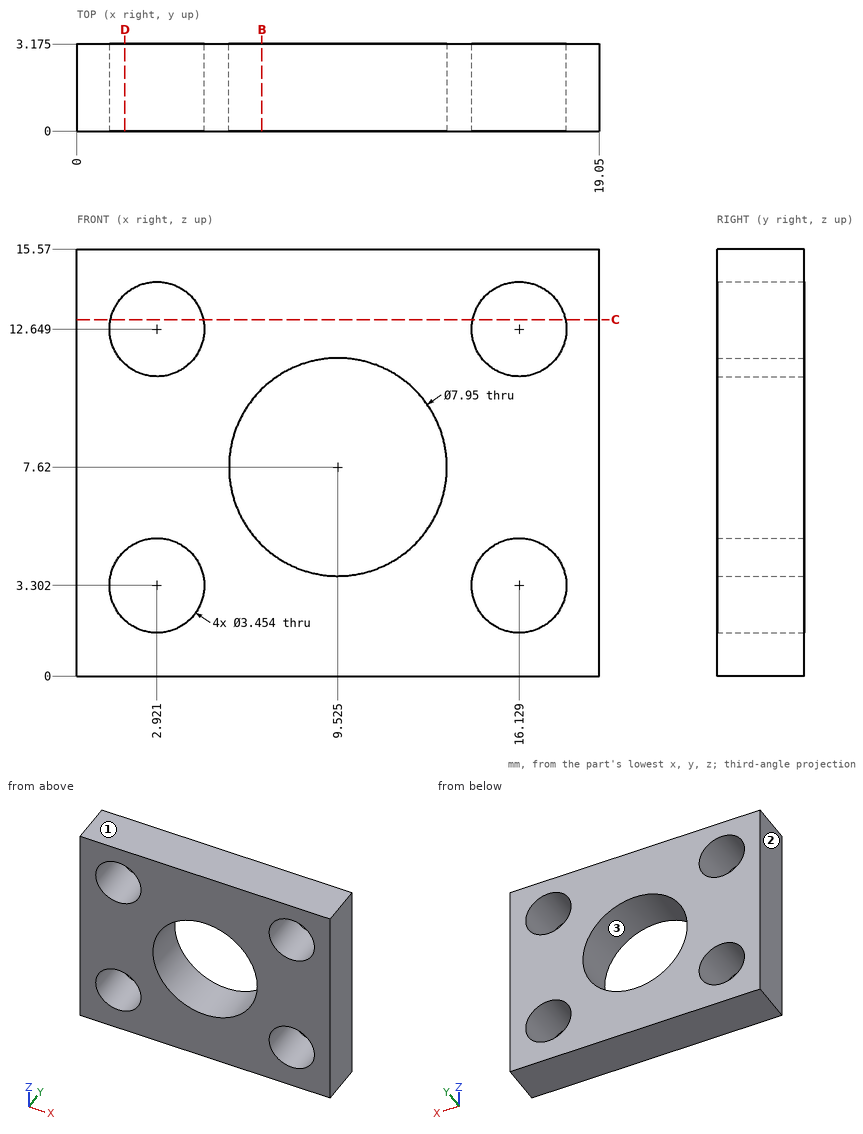
Verification items for this drawing (mm, ordinates from the low corner). Give positions to 0.01 mm unless a question says otherwise; leave off trailing zeros. Order: outer loops, then holes, each group sorted by start corner. A loop starts at its lowest first (then second) coordinate and runs counter-clockwise, first axis right, second up.
1) Cross-section at B-B (x = 6.75). Record the boundary of the cut face in (y, z) (1 decimal).
Results are:
outline: (0, 0) - (3.2, 0) - (3.2, 4.8) - (0, 4.8) - close; (0, 10.5) - (3.2, 10.5) - (3.2, 15.6) - (0, 15.6) - close
2) Cross-section at C-C (z = 13). Give the number of separate pieces and of enclosed holes in the cut face, then the cut area to 3 significant figures.
Results are:
separate pieces: 3
enclosed holes: 0
area: 39.0 mm2
3) Cross-section at D-D (x = 1.75). Record the boundary of the cut face in (y, z) (1 decimal), then the cut area to 3 significant figures.
Results are:
outline: (0, 0) - (3.2, 0) - (3.2, 2) - (0, 2) - close; (0, 4.6) - (3.2, 4.6) - (3.2, 11.4) - (0, 11.4) - close; (0, 13.9) - (3.2, 13.9) - (3.2, 15.6) - (0, 15.6) - close
area: 33.3 mm2
4) Gauge pin test, flat end, axial feed: pin 1 (7 mm diameter, centred on x = 9.525, z = 7.62, fed in from +Y). Record the tip position at first contact, or that the pin passes through.
Results are:
pin 1: passes through
5) Draft check along X on the marked faces 1, 2 and 3. Enter one of: released by +X, released by -X, zero draft, split by the parting line, or undercut.
Results are:
face 1: zero draft
face 2: released by -X
face 3: undercut
6) Material ranges on probe 1 along Z at (x, y) = (16, 2.7) (1 decimal); probe 2 along X at (y, z) = (0.95, 3); probe 3 along Z at (x, y) = (14.75, 2.5) (1 decimal), recorded low to high.
Results are:
probe 1: z = 0 to 1.6, 5 to 10.9, 14.4 to 15.6
probe 2: x = 0 to 1.22, 4.62 to 14.43, 17.83 to 19.05
probe 3: z = 0 to 2.3, 4.3 to 11.6, 13.7 to 15.6
